Verification items for this drawing (mm, ordinates from the low corner). A direction names the side the tool comes from. Round coordinates to 2 decimals unless told otherwise and drop trailing zeros. Order: outer loops, then holes, each group sorted by start corner. A loop starts at its lowest first (then second) coordinate and runs counter-clockwise, first axis right, second up.
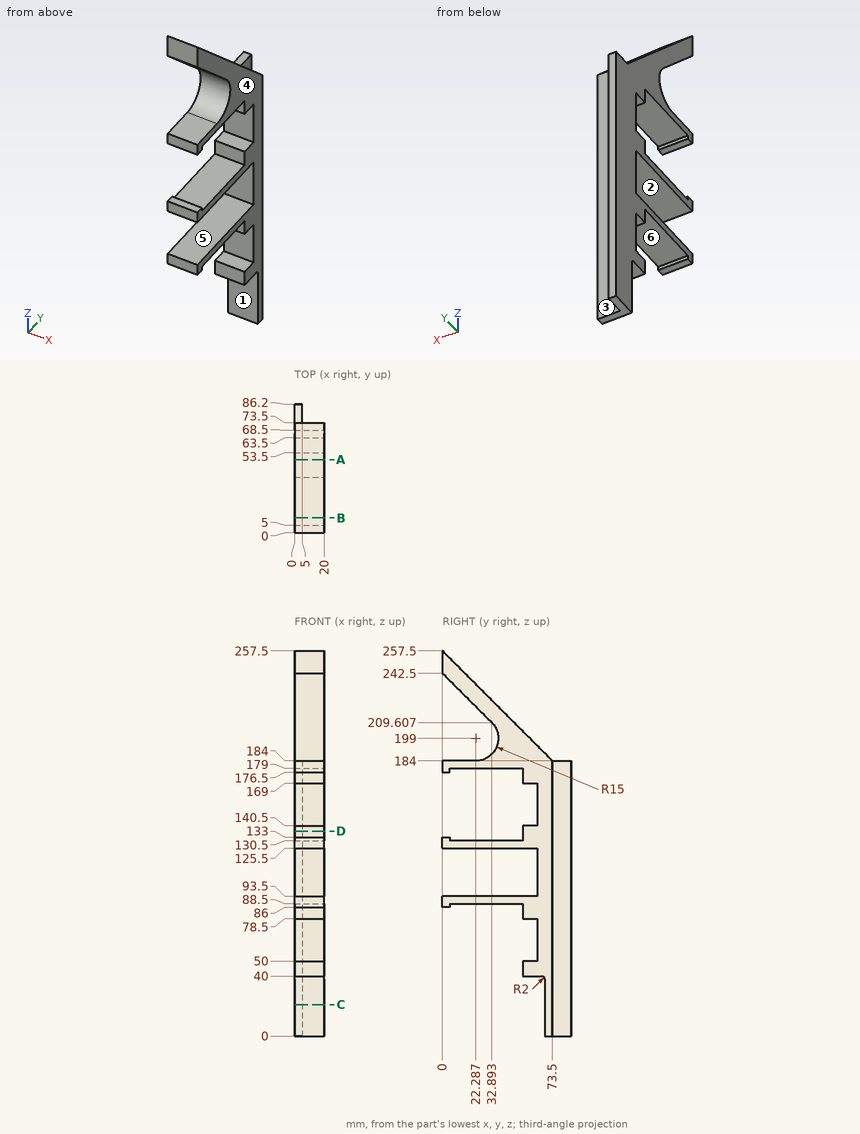
Item 1: Sectioned sample at A-A (y = 49). Record the cut outline in (x, z), and give its area (3 significant figures).
Answer:
outline: (0, 88.5) - (20, 88.5) - (20, 93.5) - (0, 93.5) - close; (0, 125.5) - (20, 125.5) - (20, 130.5) - (0, 130.5) - close; (0, 179) - (20, 179) - (20, 208.5) - (0, 208.5) - close
area: 790 mm2
Item 2: Access from +Z, -Z, +X, -X, +Y, -Y to the whole of each face (thin tool, end or side, straight path). Record for the marked faces 1, 2 and 3.
Answer:
face 1: -Z, +X, -X, -Y
face 2: +X, -X, -Y
face 3: +Z, -Z, +X, +Y
Item 3: Sectioned sample at D-D (z = 137). Record the cut outline in (x, y).
Answer:
outline: (0, 53.5) - (20, 53.5) - (20, 73.5) - (5, 73.5) - (5, 86.2) - (0, 86.2) - close
Item 4: Sectioned sample at B-B (y = 10). Record the cut outline in (x, z).
Answer:
outline: (0, 88.5) - (20, 88.5) - (20, 93.5) - (0, 93.5) - close; (0, 125.5) - (20, 125.5) - (20, 130.5) - (0, 130.5) - close; (0, 179) - (20, 179) - (20, 184) - (0, 184) - close; (0, 232.5) - (20, 232.5) - (20, 247.5) - (0, 247.5) - close
Item 5: Scan lines: line 1 along Z through (x, y) = (6.75, 57.5); line 2 along Z through (x, y) = (19.25, 8); line 3 along Z through (x, y) = (6.75, 53). Record each from-to range of solid material in increasing order.
Answer:
line 1: z = 40 to 50, 78.5 to 93.5, 125.5 to 140.5, 169 to 200
line 2: z = 88.5 to 93.5, 125.5 to 130.5, 179 to 184, 234.5 to 249.5
line 3: z = 88.5 to 93.5, 125.5 to 130.5, 179 to 204.5
Item 6: Release check for a two-part mould opening along Z. For the marked faces 4, 5 and 6 record: released by +Z, released by -Z, zero draft, split by the parting line, or undercut.
Answer:
face 4: zero draft
face 5: undercut
face 6: released by -Z
Item 7: Go/stop test with flat-tipped pins: P1, Ø12, axis at x = 15, y = 21, coming from the +Z side; P2, Ø1.2, axis at x = 7.5, z = 132, coming from the +Y side; P3, Ø8, axis at x = 14.5, y = 57, coming from the -Z side. Record where each tip stops, or that it passes through.
Answer:
P1: stops at z = 242.5
P2: stops at y = 73.5
P3: stops at z = 40
Item 8: Sectioned sample at C-C (z = 21). Record the cut outline in (x, y).
Answer:
outline: (0, 68.5) - (20, 68.5) - (20, 73.5) - (5, 73.5) - (5, 86.2) - (0, 86.2) - close
